Geometry: see drawing. Coordinates: mm, zero at the bounding-box minimum. A direction names the side the tool comes from. Round coordinates to 2 decimals unless told otherwise and drop trailing zeros. Loops run counter-clockwise (first coordinate to the right, second up) from the corner with the lowest first, then second, coordinate; pieces in that order, holes last.
(1) Section A-A, the plane x = 23. Return the cut outline in (y, z) (1 decimal).
(2) Mould query, pull axis Z, two halves, no side actions, for the marked faces 3, 4, 5 and 6. Classes: pulls with the +Z half, pulls with the -Z half, needs draft (parallel to the pull), parting line crosses it, or undercut.
(3) Section D-D, the plane x = 57. Return the cut outline in (y, z) (1 decimal).
(4) Material intervals for probe 1 along Z at (x, y) = (23.5, 19); probe 2 along Y at (x, z) = (1.05, 27.9) (1 decimal); probe 3 along X at (y, z) = (34, 48), sorted ascending.
(5) Set-up query: the marked faces 1 and 2. Return all of +Z, -Z, +X, -X, +Y, -Y with unobstructed straight access to the full face (end or side cutting, diameter ignored); none if empty.
(6) Section B-B, the plane z = 27.9. Return the cut outline in (x, y) (1 decimal).
(7) First-contact query: pin 1 Ø9.5 at (x, y) = (55.88, 14) entering from -Z; pin 2 Ø9 at (y, z) = (29.5, 17.5) entering from +X; pin 3 Ø8 at (y, z) = (33.21, 27.9) entering from -X. Flat tips, straight axial feed; report the tip coordinate or a pass-through.
(8) Section C-C, the plane y = 15.5. Return the cut outline in (x, z) (1 decimal).
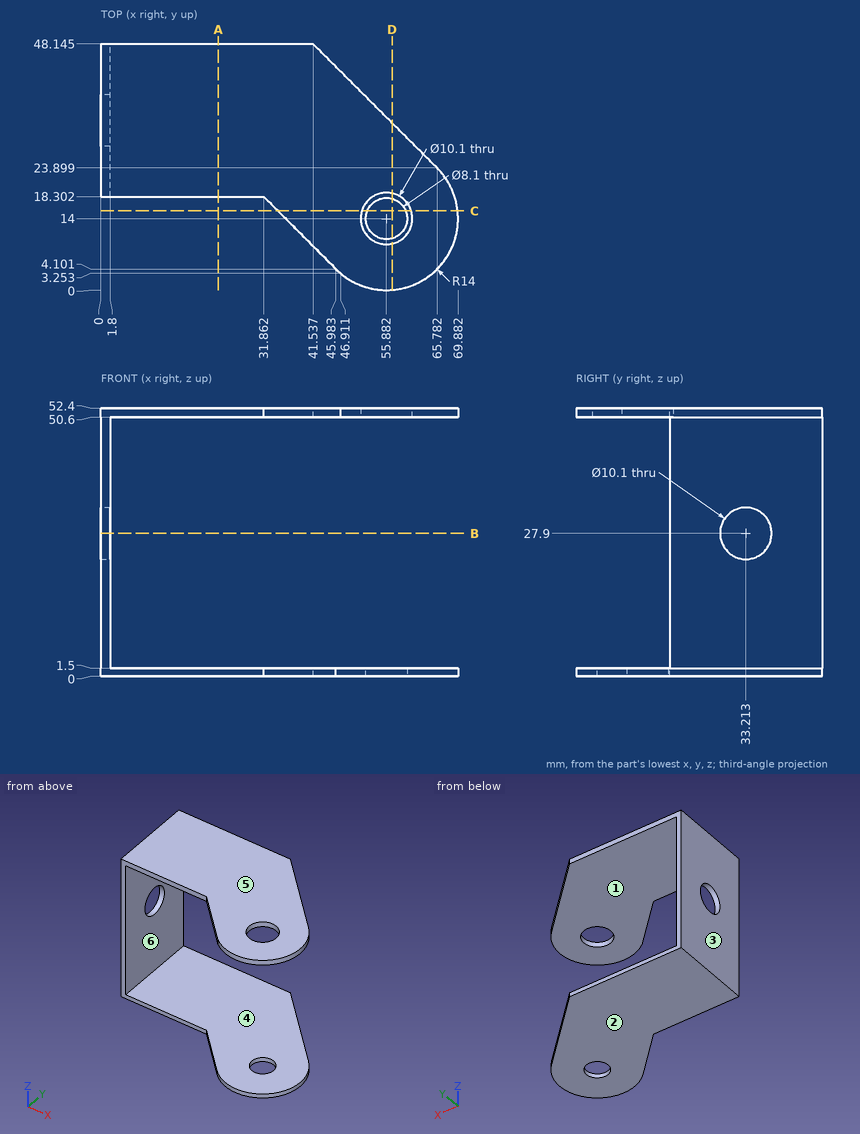
Output values:
1. outline: (18.3, 0) - (48.1, 0) - (48.1, 1.5) - (18.3, 1.5) - close; (18.3, 50.6) - (48.1, 50.6) - (48.1, 52.4) - (18.3, 52.4) - close
2. face 3: needs draft
2. face 4: undercut
2. face 5: pulls with the +Z half
2. face 6: undercut
3. outline: (0, 0) - (10.1, 0) - (10.1, 1.5) - (0, 1.5) - close; (0, 50.6) - (9.1, 50.6) - (9.1, 52.4) - (0, 52.4) - close; (17.9, 0) - (32.7, 0) - (32.7, 1.5) - (17.9, 1.5) - close; (18.9, 50.6) - (32.7, 50.6) - (32.7, 52.4) - (18.9, 52.4) - close
4. probe 1: z = 0 to 1.5, 50.6 to 52.4
4. probe 2: y = 18.3 to 28.2, 38.3 to 48.1
4. probe 3: x = 0 to 1.8
5. face 1: +X, +Y, -Y
5. face 2: -Z, +X, -X, +Y, -Y
6. outline: (0, 18.3) - (1.8, 18.3) - (1.8, 28.2) - (0, 28.2) - close; (0, 38.3) - (1.8, 38.3) - (1.8, 48.1) - (0, 48.1) - close
7. pin 1: stops at z = 0
7. pin 2: stops at x = 1.8
7. pin 3: passes through
8. outline: (34.6, 0) - (52.1, 0) - (52.1, 1.5) - (34.6, 1.5) - close; (34.7, 50.6) - (51.1, 50.6) - (51.1, 52.4) - (34.7, 52.4) - close; (59.6, 0) - (69.8, 0) - (69.8, 1.5) - (59.6, 1.5) - close; (60.7, 50.6) - (69.8, 50.6) - (69.8, 52.4) - (60.7, 52.4) - close
